Input: dimensioned drawing with shaded views. Units: mm. Origin: part minimum x, y, z. A direction names the side the tool comes from. Round coordinates to 2 decimals unless told otherwise and drop trailing zeros. Write each loop counter-clockwise with the first axis right and the second up, starting at its lowest first coordinate (ties: lowest second). Pieces come first, ordered by that corner, then holes. Notation, with made-up numbers: (-27, -1.75) - (9, -1.75) arc R3 cw to (9, 3.25) - close; hole circle Ø11 at (77.5, 40.25). An arc over 180 degrees is marked (long way). Use one line per item in the form item = value.
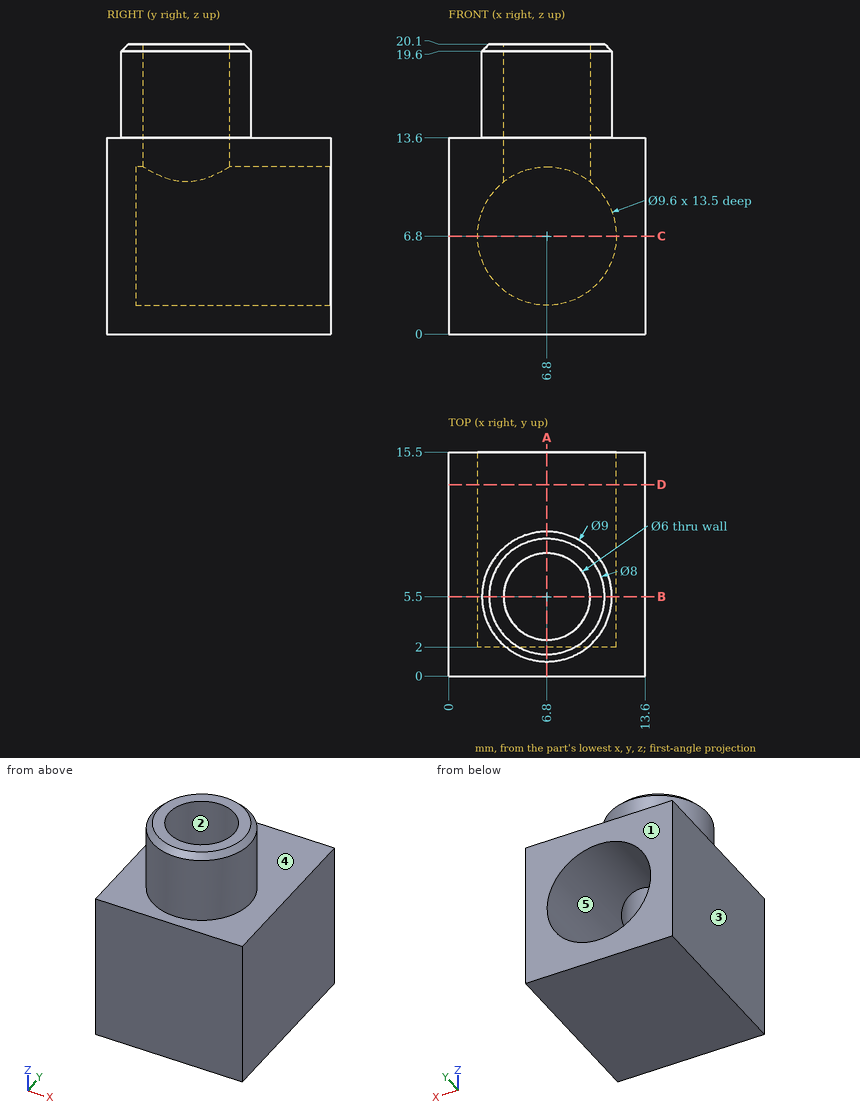
(1) Material intervals for L1, parallel to Y at x = 6.8, z = 15; L2, parallel to X at y = 5.5, z = 13.5; L3, parallel to Z at x = 6.75, y = 6.75, sorted ascending.
Derived:
L1 = 1 to 2.5, 8.5 to 10
L2 = 0 to 3.8, 9.8 to 13.6
L3 = 0 to 2
(2) Cut plane A-A on x = 6.8. Output: boundary loops of the cut face in (y, z), then the cut area to 4 significant figures.
Derived:
outline = (0, 0) - (15.5, 0) - (15.5, 2) - (2, 2) - (2, 11.6) - (2.5, 11.6) - (2.5, 20.1) - (1.5, 20.1) - (1, 19.6) - (1, 13.6) - (0, 13.6) - close; (8.5, 11.6) - (15.5, 11.6) - (15.5, 13.6) - (10, 13.6) - (10, 19.6) - (9.5, 20.1) - (8.5, 20.1) - close
area = 88.45 mm^2
(3) First-contact query: pin 1 Ø7 at (x, y) = (6.8, 5.5) entering from +Z; pin 2 Ø1 at (x, y) = (11.5, 8.5) entering from +Z; pin 3 Ø6 at (y, z) = (12, 18) entering from -X; pin 4 Ø1.5 at (x, y) = (7, 7) entering from +Z. Flat tips, straight axial feed; report the tip coordinate or a pass-through.
Derived:
pin_1 = 20.1
pin_2 = 13.6
pin_3 = 3.97
pin_4 = 2.09
(4) Cut plane C-C on z = 6.8. Output: boundary loops of the cut face in (x, y).
Derived:
outline = (0, 0) - (13.6, 0) - (13.6, 15.5) - (11.6, 15.5) - (11.6, 2) - (2, 2) - (2, 15.5) - (0, 15.5) - close
(5) Cut plane D-D on y = 13.25. Output: boundary loops of the cut face in (x, z).
Derived:
outline = (0, 0) - (13.6, 0) - (13.6, 13.6) - (0, 13.6) - close; hole circle Ø9.6 at (6.8, 6.8)
(6) Access query for the marked faces 1 and 2. Directions: +Z, -Z, +X, -X, +Y, -Y. A direction counts if a zero-diameter tool reaches every point of the face in a straight line with its end or side. Return the directions, or none.
Derived:
face_1 = +Z, -Z, +X, -X, +Y
face_2 = +Z
(7) Cut plane B-B on y = 5.5. Output: boundary loops of the cut face in (x, z), then the cut area to 3 significant figures.
Derived:
outline = (0, 0) - (13.6, 0) - (13.6, 13.6) - (11.3, 13.6) - (11.3, 19.6) - (10.8, 20.1) - (9.8, 20.1) - (9.8, 10.55) arc R4.8 cw (long way) to (3.8, 10.55) - (3.8, 20.1) - (2.8, 20.1) - (2.3, 19.6) - (2.3, 13.6) - (0, 13.6) - close
area = 118 mm^2
(8) Draft query along Z for the marked faces 3, 4 and 5. Return one class per face: released by +Z, released by -Z, zero draft, split by the parting line, or undercut.
Derived:
face_3 = zero draft
face_4 = released by +Z
face_5 = undercut
